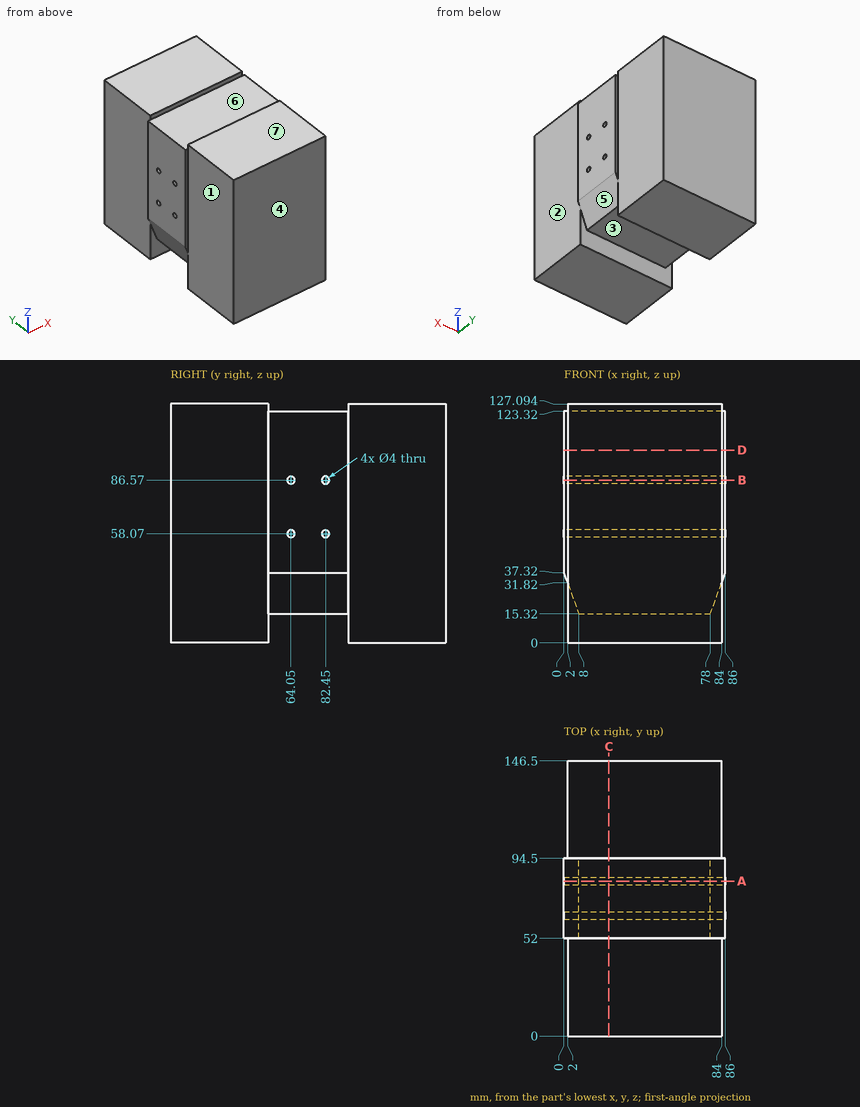
Design review of the part shown in the three views and the two pictorial views. Dimensions are in mm from the part's minimum x, y and z. A direction names the side the tool comes from. Give positions to 0.01 mm unless a question says otherwise; leave off trailing zeros. Write each loop counter-clockwise with the first axis right and the second up, starting at its lowest first coordinate (ties: lowest second). Pieces come first, ordered by that corner, then holes.
(1) Add section D-D (z = 102.5). Give the boundary of the cut face in (x, y).
Checked values:
outline: (0, 52) - (2, 52) - (2, 0) - (84, 0) - (84, 52) - (86, 52) - (86, 94.5) - (84, 94.5) - (84, 146.5) - (2, 146.5) - (2, 94.5) - (0, 94.5) - close
(2) Wall thickness on line 1 along Y through (x, z) = (33, 58); line 2 along Z through (x, y) = (26, 64.05); line 3 along X through (y, z) = (101, 122): over which ranges is each line inside the solid? List them lowest first.
Checked values:
line 1: y = 0 to 62.05, 66.05 to 80.45, 84.45 to 146.5
line 2: z = 15.32 to 56.07, 60.07 to 84.57, 88.57 to 123.32
line 3: x = 2 to 84
(3) Tool access review of the marked faces 1, 2 and 3: name each direction out of +Z, -Z, +X, -X, +Y, -Y from which nothing blocks a thin tool from reaching the whole face with its end or side.
Checked values:
face 1: +Z, -Z, -X, -Y
face 2: +Z, -Z, +X, -Y
face 3: -Z, +X, -X
(4) Mouldability with a two-part tool opening along Y and no side actions: class the marked faces 4, 5, 6 and 7 as +Y half, -Y half, draft (parallel to the pull), parting line (faces both ways), or undercut.
Checked values:
face 4: -Y half
face 5: undercut
face 6: undercut
face 7: draft
(5) Add section B-B (z = 86.57). Give the boundary of the cut face in (x, y), and give its area (3 significant figures).
Checked values:
outline: (0, 52) - (2, 52) - (2, 0) - (84, 0) - (84, 52) - (86, 52) - (86, 62.05) - (0, 62.05) - close; (0, 66.05) - (86, 66.05) - (86, 80.45) - (0, 80.45) - close; (0, 84.45) - (86, 84.45) - (86, 94.5) - (84, 94.5) - (84, 146.5) - (2, 146.5) - (2, 94.5) - (0, 94.5) - close
area: 11,500 mm2
(6) Add section A-A (y = 82.45). Give the boundary of the cut face in (x, z).
Checked values:
outline: (0, 37.32) - (8, 15.32) - (78, 15.32) - (86, 37.32) - (86, 56.07) - (0, 56.07) - close; (0, 60.07) - (86, 60.07) - (86, 84.57) - (0, 84.57) - close; (0, 88.57) - (86, 88.57) - (86, 123.32) - (0, 123.32) - close
(7) Clearance check with flat-ended pins moving along their axes: pin 1 Ø5 at (y, z) = (82.45, 86.57) entering from +X; pin 2 Ø3 at (y, z) = (69.5, 14) entering from +X; pin 3 Ø6 at (x, y) = (51.5, 72.5) entering from +Z; pin 4 Ø1 at (y, z) = (117.5, 112.5) entering from -X. State where each tip first meets the part, or that it passes through.
Checked values:
pin 1: stops at x = 86
pin 2: stops at x = 78.07
pin 3: stops at z = 123.32
pin 4: stops at x = 2
(8) Add section C-C (x = 24). Give the boundary of the cut face in (y, z).
Checked values:
outline: (0, 0) - (52, 0) - (52, 15.32) - (94.5, 15.32) - (94.5, 0) - (146.5, 0) - (146.5, 127.09) - (94.5, 127.09) - (94.5, 123.32) - (52, 123.32) - (52, 127.09) - (0, 127.09) - close; hole circle Ø4 at (64.05, 58.07); hole circle Ø4 at (64.05, 86.57); hole circle Ø4 at (82.45, 58.07); hole circle Ø4 at (82.45, 86.57)
